Solid Edge part; units mm, degrees
sketch "Sketch1" plane through (0, 0, 0) normal (0, -1, 0) x (1, 0, 0)
  line L0 (-1.5875, -36.478) -> (-1.5875, -38.0669)
  arc A0 (-1.5875, -38.0669) -> (-1.5875, 38.0669) centre (0, 0) cw
  line L1 (-1.5875, 38.0669) -> (-1.5875, 36.478)
  arc A1 (-1.5875, -36.478) -> (-1.5875, 36.478) centre (0, 0) cw
extrude "Protrusion1" add sketch "Sketch1" along normal mid plane 127
sketch "Sketch2" plane through (0, 0, 0) normal (0, -1, 0) x (1, 0, 0)
  circle A0 centre (0, 49.1794) radius 6.35
  line L0 (-25.4, 41.2419) -> (-5.4073, 54.9902)
  line L1 (-1.5875, 38.0669) -> (4.7625, 42.8294)
  line L2 (-25.4, 41.2419) -> (-25.4, 28.3981)
  arc A1 (-5.4073, 54.9902) -> (4.7625, 42.8294) centre (0, 49.1794) cw
  arc A2 (-1.5875, 38.0669) -> (-25.4, 28.3981) centre (0, 0) ccw
extrude "ExtrudedProtrusion_2" add sketch "Sketch2" along normal mid plane 25.4
sketch "Sketch3" plane through (-19.8437, -63.5, 0) normal (0, -1, 0) x (0, 0, -1)
  line L0 (-40.9984, 16.4824) -> (-38.1, 19.8437)
  line L1 (-44.6712, 18.9824) -> (-40.9984, 16.4824)
  line L2 (-44.6712, 18.9824) -> (-46.598, 14.9833)
  line L3 (-50.7924, 16.4486) -> (-46.598, 14.9833)
  line L4 (-50.7924, 16.4486) -> (-51.6195, 12.0873)
  line L5 (-56.0501, 12.418) -> (-51.6195, 12.0873)
  line L6 (-56.0501, 12.418) -> (-55.7213, 7.9911)
  line L7 (-60.0868, 7.165) -> (-55.7213, 7.9911)
  line L8 (-60.0868, 7.165) -> (-58.6244, 2.9737)
  line L9 (-62.6277, 1.0467) -> (-58.6244, 2.9737)
  line L10 (-62.6277, 1.0467) -> (-60.1312, -2.6239)
  line L11 (-63.5, -5.5205) -> (-60.1312, -2.6239)
  line L12 (-63.5, -5.5205) -> (-60.1392, -8.4207)
  line L13 (-60.1392, -8.4207) -> (-28.1345, -5.8479)
  line L14 (-36.478, 18.2562) -> (-38.0669, 18.2562)
  line L15 (-38.1, 19.8437) -> (-36.478, 18.2562)
  arc A0 (-38.0669, 18.2563) -> (-28.1345, -5.8479) centre (0, 19.8437) ccw
extrude "ExtrudedProtrusion_3" add sketch "Sketch3" against normal blind 3.175
Work out the finished part from the listing and answer in its coordinate system (mm). A direction names the side the tool comes from. Coordinates: 2 decimals unless noted, no trailing zeros. Loops run counter-clockwise (first coordinate to the right, second up) from the corner with the lowest first, then second, coordinate; pieces in that order, holes last.
1) Section A-A (x = -14.5) is taken. Give the vertices of the cut face in (y, z) (3 decimals).
Results:
outline: (-63.5, -35.233) - (63.5, -35.233) - (63.5, -33.51) - (-63.5, -33.51) - close; (-63.5, 33.51) - (63.5, 33.51) - (63.5, 35.233) - (12.7, 35.233) - (12.7, 48.737) - (-12.7, 48.737) - (-12.7, 35.233) - (-60.325, 35.233) - (-60.325, 59.451) - (-63.5, 59.451) - close
2) Section C-C (z = 0) is taken. Give the vertices of the cut face in (x, y), plus the area to 3 significant figures.
Results:
outline: (-38.1, -63.5) - (-36.51, -63.5) - (-36.51, 63.5) - (-38.1, 63.5) - close
area: 202 mm2
3) For a pull along X with two mould halves and no side action, classify faces 5 (the flat face through (-2.83, -61.93, 45.62)), 6 (the flat face through (-17.847, -61.935, 60.654)), 7 (the flat face through (-27, -61.9, 44.4)) as +X half, -X half, draft (parallel to the pull), parting line (faces both ways), or undercut.
Results:
face 5: +X half
face 6: undercut
face 7: -X half
4) Section B-B (y = -47) is taken. Give the vertices of the cut face in (x, z).
Results:
outline: (-1.59, -38.07) - (-1.59, -36.48) arc R36.51 cw to (-1.59, 36.48) - (-1.59, 38.07) arc R38.1 ccw to start
5) Flat-ended cylindrical pins translate along their axes: pin 1 (1.5 mm diameter, centred on x = -12.5, y = 20.5, fed in from -Z); pin 2 (0.5 mm diameter, centred on y = 2.5, z = 37.5, fed in from +X); pin 3 (10 mm diameter, centred on y = 14, z = -12, fed in from +X); pin 4 (16.5 mm diameter, centred on x = 0, z = 49.18, fed in from -Y). Find the tip coordinate at first contact, or state that the pin passes through.
Results:
pin 1: stops at z = -36.24
pin 2: stops at x = -1.59
pin 3: stops at x = -32.31
pin 4: stops at y = -63.5
6) For faces 1 (the cylindrical face through (-0.827, 0.178, 42.883)), 2 (the flat face through (-12, -12.7, 43)), 3 (the flat face through (-2, -62, 43)), 4 (the flat face through (-15.54, 0.18, 48.02)), determine the directions among +Z, -Z, +X, -X, +Y, -Y from which every point of the face is accessible in a straight line to the end or side of a thin tool.
Results:
face 1: +Y
face 2: +Z, -X
face 3: +X, -Y
face 4: +Z, -X, +Y
7) Consider probe 1 along Y at (x, z) = (-10.5, 37.5) (3 decimals); probe 2 along Z at (x, y) = (0, -1.75); probe 3 along Z at (x, y) = (-2.5, -2). Determine where each line is inside the solid, lowest interval first.
Results:
probe 1: y = -63.5 to -60.325, -12.7 to 12.7
probe 2: z = 39.26 to 42.83, 55.53 to 57.12
probe 3: z = -38.02 to -36.43, 36.43 to 43.34, 55.02 to 56.71
